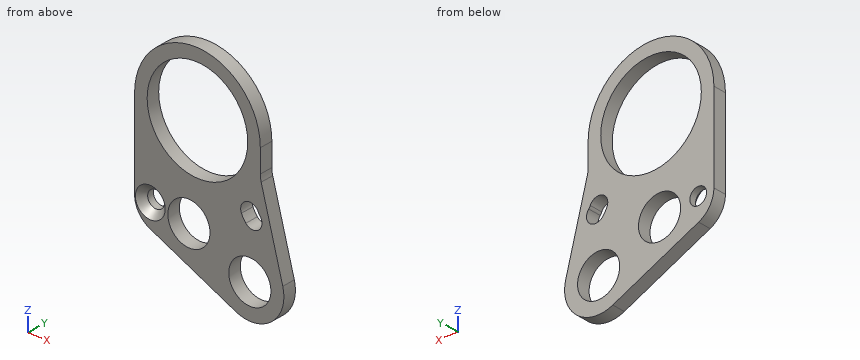
Autodesk Inventor part; units mm, degrees
ref_plane "YZ Plane" through (0, 0, 0) normal (1, 0, 0) x (0, 1, 0)
ref_plane "XZ Plane" through (0, 0, 0) normal (0, 1, 0) x (-1, 0, 0)
ref_plane "XY Plane" through (0, 0, 0) normal (0, 0, 1) x (1, 0, 0)
sketch "Sketch1" plane through (0, 0, 0) normal (0, 1, 0) x (-1, 0, 0)
  circle A0 centre (0, 0) radius 1.6
  circle A1 centre (10, 11.472032) radius 12
  line L0 (0, 0) -> (10, 11.472032) construction
  line L1 (0, 0) -> (4, 0) construction
  circle A2 centre (0, 0) radius 4
  circle A3 centre (0, -11.440846) radius 6.5
  line L2 (10, 11.472032) -> (0, -11.440846) construction
  line L3 (0, 0) -> (0, -11.440846) construction
  line L4 (0, 0) -> (0, -4) construction
  line L5 (22, 11.472032) -> (22, -8.527968)
  line L6 (22, -8.527968) -> (2.703128, -17.352115)
  line L7 (-2, 11.472032) -> (-2, 6.472032)
  line L8 (-2, 6.472032) -> (-6.285281, -9.783969)
  circle A4 centre (10, 11.472032) radius 9.6
  line L9 (10, 11.472032) -> (17.5, 11.472032) construction
  circle A5 centre (17.5, 11.472032) radius 1.075
  circle A6 centre (6.25, 17.967223) radius 1.075
  circle A7 centre (6.25, 4.976842) radius 1.075
  circle A8 centre (10, 11.472032) radius 6.1
  circle A9 centre (0, -11.440846) radius 4.025
  circle A10 centre (10, 11.472032) radius 10
  circle A11 centre (0, -11.440846) radius 5
  circle A12 centre (11.624641, -6.20346) radius 7.75
  circle A13 centre (11.624641, -6.20346) radius 4.025
  circle A14 centre (19, -5.527968) radius 1.6
  dimension "d5" = 8
  dimension "d0" = 3.2
  dimension "d1" = 24
  dimension "d2" = 4
  dimension "d4" = 10
  dimension "d6" = 13
  dimension "d7" = 25
  dimension "d8" = 17.5
  dimension "d12" = 0
  dimension "d13" = 20
  dimension "d14" = 5
  dimension "d17" = 19.2
  dimension "d19" = 7.5
  dimension "d20" = 2.15
  dimension "d23" = 360
  dimension "d25" = 12.2
  dimension "d26" = 8.05
  dimension "d38" = 20
  dimension "d39" = 10
  dimension "d40" = 15.5
  dimension "d41" = 8.05
  dimension "d42" = 3.2
  dimension "d43" = 3
  dimension "d44" = 3
sketch "Sketch1 outline for Extrusion1" plane through (0, 0, 0) normal (0, 1, 0) x (-1, 0, 0)
  line L0 (-2, 11.472032) -> (-2, 6.472032)
  line L1 (-2, 6.472032) -> (-6.285281, -9.783969)
  arc A0 (-6.285281, -9.783969) -> (2.703128, -17.352115) centre (0, -11.440846) ccw
  line L2 (2.703128, -17.352115) -> (22, -8.527968)
  line L3 (22, -8.527968) -> (22, 11.472032)
  arc A1 (22, 11.472032) -> (-2, 11.472032) centre (10, 11.472032) ccw
  circle A2 centre (0, -11.440846) radius 4.025
  circle A3 centre (11.624641, -6.20346) radius 4.025
  circle A4 centre (10, 11.472032) radius 9.6
extrude "Extrusion1" add sketch "Sketch1 outline for Extrusion1" against normal blind 2.5
fillet "Fillet1" radius 5 2 edges at (-22, -1.25, -8.528) (2, -1.25, 6.472)
sketch "Sketch2" plane through (0, -2.5, 0) normal (0, -1, 0) x (1, 0, 0)
  point P0 (0, 0)
  point P1 (-19, -5.527968)
hole "Hole3" at (-19, -2.5, -5.527968) direction (0, 1, 0) diameter 3.2 end through all countersink diameter 5.7 countersink angle 90
sketch "Sketch3" plane through (0, 0, 0) normal (0, 1, 0) x (1, 0, 0)
  circle A0 centre (0, 0) radius 1.75 construction
  line L0 (2, -1.472032) -> (3.318061, -1.472032) construction
  line L1 (6.285281, 9.783969) -> (2.165168, -5.845474)
  arc A1 (0.568061, 0.897337) -> (0, 0) centre (3.318061, -1.472032) ccw construction
  arc A2 (-0.757721, 2.039616) -> (-1.599646, 0.709671) centre (3.318061, -1.472032) ccw
  arc A3 (1.893843, -0.244942) -> (1.599646, -0.709671) centre (3.318061, -1.472032) ccw
  arc A4 (1.893843, -0.244942) -> (-0.757721, 2.039616) centre (0.568061, 0.897337) ccw
  arc A5 (-1.599646, 0.709671) -> (1.599646, -0.709671) centre (0, 0) ccw
  line L2 (2, -1.472032) -> (2, -6.472032) construction
  point P0 (2, -6.472032)
  dimension "d68" = 2.75
  dimension "d69" = 5
extrude "Extrusion3" cut sketch "Sketch3" against normal blind 2.5
properties part number "Dribbler Bracket B"
Build history of the part. All positions in model axes, mm. Round coordinates to 2 decimals unless told otherwise and drop trailing zeros. Write each loop counter-clockwise with the first axis right and the second up, starting at its lowest first coordinate (ties: lowest second). Pieces come first, ordered by that corner, then holes.
1) Band-saw the part on C-C, the plane x = -9.75. List the corners of the cut face in (y, z).
2) Drill centre lines: probe 1 along X at (y, z) = (-0.55, -8) (3 decimals); probe 2 along Z at (x, y) = (-9.25, -2.05); probe 3 along Z at (x, y) = (-9.5, -1.35). Where is each one in solid material? Low to high.
3) Band-saw the part on B-B, the plane y = -2.05. List the corners of the cut face in (x, z) (3 decimals), and give its area (3 significant figures).
4) Band-saw the part on D-D, the plane z = -9. List the corners of the cut face in (x, y).
5) Band-saw the part on A-A, the plane z = -14. List the corners of the cut face in (x, y) (3 decimals).
6) Pin check, flat tips, straight feed: pin 1 (1.9 mm diameter, centred on x = -19, z = -5.53, fed in from +Y); pin 2 (1.5 mm diameter, centred on y = -0.5, z = -12.5, fed in from -X). Stop position of each tip, or through.
Ans:
1. outline: (-2.5, -14.13) - (0, -14.13) - (0, -9.77) - (-2.5, -9.77) - close; (-2.5, -2.64) - (0, -2.64) - (0, 1.88) - (-2.5, 1.88) - close; (-2.5, 21.07) - (0, 21.07) - (0, 23.47) - (-2.5, 23.47) - close
2. probe 1: x = -21.219 to -15.226, -8.023 to -2.088, 2.088 to 5.815
2. probe 2: z = -14.36 to -9.45, -2.95 to 1.9, 21.04 to 23.45
2. probe 3: z = -14.24 to -9.62, -2.78 to 1.89, 21.06 to 23.46
3. outline: (-22, -5.316) arc R5 ccw to (-19.079, -9.864) - (-2.703, -17.352) arc R6.5 ccw to (6.285, -9.784) - (2.165, 5.845) arc R5 cw to (2, 7.12) - (2, 11.472) arc R12 ccw to (-22, 11.472) - close; hole circle Ø4.8 at (-19, -5.528); hole circle Ø19.2 at (-10, 11.472); hole circle Ø8.05 at (-11.625, -6.203); hole circle Ø8.05 at (0, -11.441); hole (-1.6, -0.71) arc R5.38 ccw to (-0.758, -2.04) arc R1.75 ccw to (1.894, 0.245) arc R1.88 cw to (1.6, 0.71) arc R1.75 ccw to start
3. area: 473 mm2
4. outline: (-20.38, -2.5) - (-14.52, -2.5) - (-14.52, 0) - (-20.38, 0) - close; (-8.73, -2.5) - (-3.2, -2.5) - (-3.2, 0) - (-8.73, 0) - close; (3.2, -2.5) - (6.08, -2.5) - (6.08, 0) - (3.2, 0) - close
5. outline: (-10.034, -2.5) - (-3.107, -2.5) - (-3.107, 0) - (-10.034, 0) - close; (3.107, -2.5) - (5.975, -2.5) - (5.975, 0) - (3.107, 0) - close
6. pin 1: passes through
6. pin 2: stops at x = -14.95
